Can you work these out from the drawing? Everything is in mm from the part's minimum corner. Coordinates: 2 decimals unless noted, no trailing zeros. Loops run counter-clockwise (first coordinate to the right, second up) from the corner with the lowest first, then second, coordinate; pieces in that order, holes last. Notation, with made-up numbers: (0.25, 56) - (55.25, 56) arc R22 ccw to (55.25, 91) - close; hole circle Ø3 at (-34, 36.25). An arc over 180 degrees is marked (long way). One line per question, with ' | ' between items. Start each with the question number.
1. Please list where these lines run through material, in increasing order: L1, parallel to X at y = 1.65, z = 115.5 (1 decimal); L2, parallel to X at y = 2, z = 53 (1 decimal); L3, parallel to X at y = 0.45, z = 71. Write a range as [from, to].
2. I'm going to push flat-ended pins straight in: P1, Ø1.6, axis at x = 127.5, y = 2, coming from the -Z side (1 decimal); P2, Ø1, axis at x = 2, y = 2.5, coming from the +Z side; P3, Ø1.6, axis at y = 1.5, z = 168, coming from the +X side (1 decimal). Where does each tip first touch, or does it pass through?
3. I want a section at B-B, the plane x = 33. Count the separate pieces of the cut face and the enclosed holes in it, then the cut area to 3 significant figures.
4. I want a section at A-A, the plane z = 64.5. Write out the boundary of the cut face in (x, y) (1 decimal).
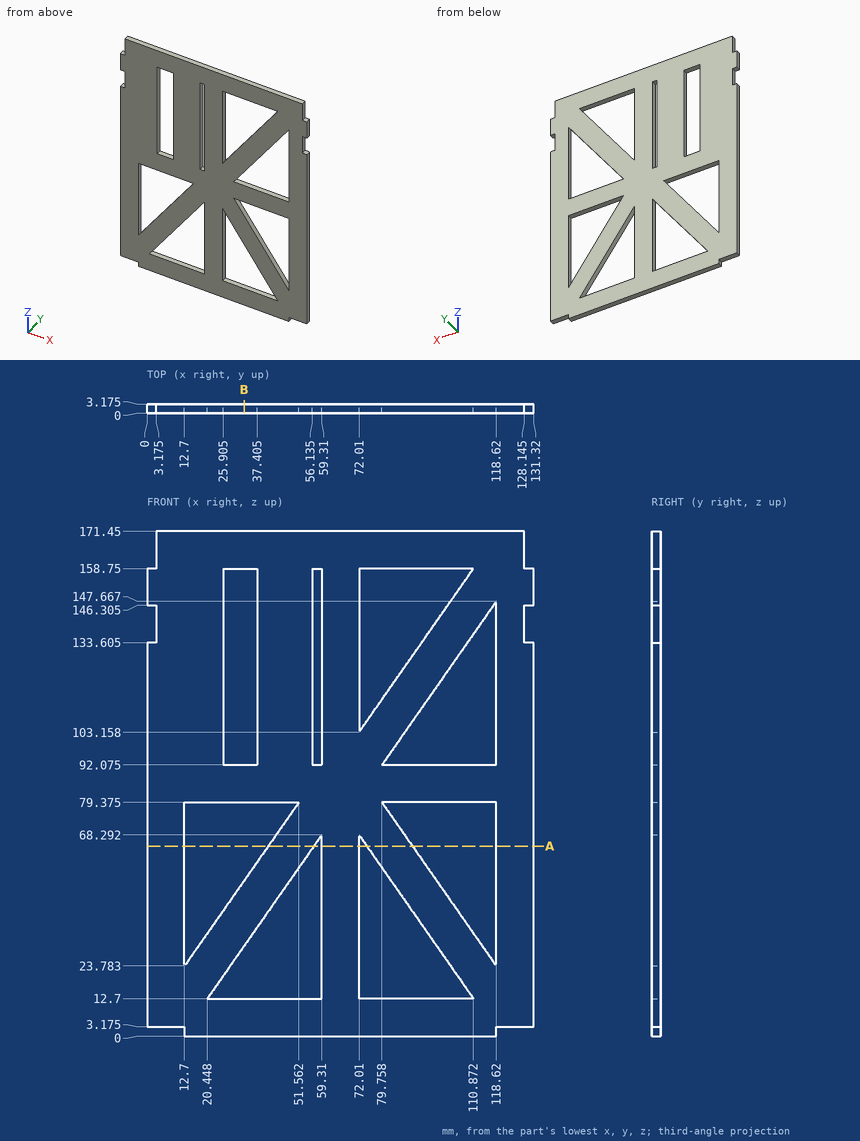
Results are:
1) L1: x = [0, 25.9], [37.4, 56.1], [59.3, 72], [80.6, 96.1], [118.6, 131.3] | L2: x = [0, 12.7], [33.1, 48.6], [59.3, 72], [82.7, 98.2], [118.6, 131.3] | L3: x = [0, 12.7], [45.71, 85.61], [118.62, 131.32]
2) P1: stops at z = 3.2 | P2: stops at z = 158.75 | P3: stops at x = 128.1
3) separate pieces: 4 | enclosed holes: 0 | area: 191 mm2
4) outline: (0, 0) - (12.7, 0) - (12.7, 3.2) - (0, 3.2) - close; (41.2, 0) - (56.7, 0) - (56.7, 3.2) - (41.2, 3.2) - close; (59.3, 0) - (72, 0) - (72, 3.2) - (59.3, 3.2) - close; (74.7, 0) - (90.2, 0) - (90.2, 3.2) - (74.7, 3.2) - close; (118.6, 0) - (131.3, 0) - (131.3, 3.2) - (118.6, 3.2) - close
